Geometry: see drawing. Coordinates: mm, zero at the bounding-box minimum. Round coordinates to 2 decimals unless told otherwise and drop trailing zeros. Write each loop counter-clockwise with the first axis right and the second up, starting at its lowest first coordinate (ties: lowest second). Pieces come first, ordered by that corner, then holes. Notation, with made-up numbers: (-31, 89) -> (25, 89) arc R19 ccw to (25, 102) -> close; hole circle Ø4 at (67, -10.75). An arc over 180 degrees is marked (long way). Use CSV: the item, a comma, the result in double quotes.
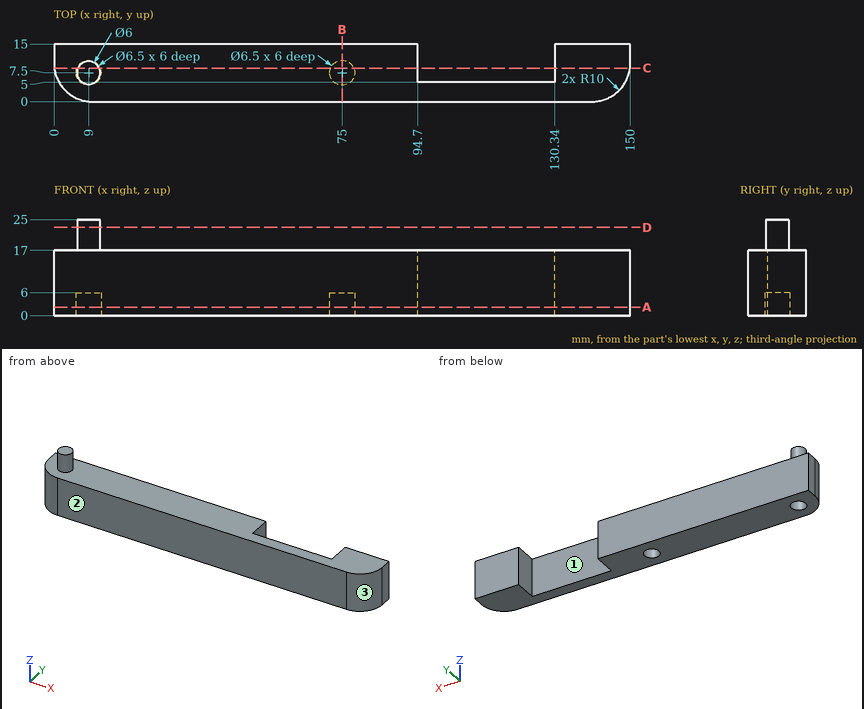
Item 1: Section query B-B on x = 75. Return the cut outline in (y, z).
Worked answers:
outline,"(0, 0) -> (4.25, 0) -> (4.25, 6) -> (10.75, 6) -> (10.75, 0) -> (15, 0) -> (15, 17) -> (0, 17) -> close"
Item 2: Section query D-D on z = 23. Return the cut outline in (x, y), plus the area to 3 significant figures.
Worked answers:
outline,"circle Ø6 at (9, 7.5)"
area,"28.3 mm²"
Item 3: Pull-direction query (X, two-part tool) for the marked faces 1, 2 and 3; classes: +X half, -X half, draft (parallel to the pull), parting line (faces both ways), or undercut.
Worked answers:
face 1,"undercut"
face 2,"draft"
face 3,"+X half"
Item 4: Section query A-A on z = 2.25. Return the cut outline in (x, y), plus the area to 3 significant figures.
Worked answers:
outline,"(0, 10) arc R10 ccw to (10, 0) -> (140, 0) arc R10 ccw to (150, 10) -> (150, 15) -> (130.34, 15) -> (130.34, 5) -> (94.7, 5) -> (94.7, 15) -> (0, 15) -> close; hole circle Ø6.5 at (9, 7.5); hole circle Ø6.5 at (75, 7.5)"
area,"1,780 mm²"
Item 5: Line query: line 1 (Y direction, x = 75, z = 1.6); line 2 (X direction, y = 12.75, z = 15.25); line 3 (Y direction, x = 9, z = 2.6). Output: solid intervals per line, ascending.
Worked answers:
line 1,"y = 0 to 4.25, 10.75 to 15"
line 2,"x = 0 to 94.7, 130.34 to 150"
line 3,"y = 0.05 to 4.25, 10.75 to 15"
Item 6: First-contact query: pin 1 Ø5 at (y, z) = (6.5, 19) entering from +X; pin 2 Ø2 at (x, y) = (8, 7) entering from -Z; pin 3 Ø8.5 at (x, y) = (75, 7.5) entering from +Z. Flat tips, straight axial feed; report the tip coordinate or a pass-through.
Worked answers:
pin 1,"stops at x = 149.8"
pin 2,"stops at z = 6"
pin 3,"stops at z = 17"
Item 7: Section query C-C on y = 8.75. Return the cut outline in (x, z).
Worked answers:
outline,"(0.08, 0) -> (6, 0) -> (6, 6) -> (12, 6) -> (12, 0) -> (72, 0) -> (72, 6) -> (78, 6) -> (78, 0) -> (94.7, 0) -> (94.7, 17) -> (11.73, 17) -> (11.73, 25) -> (6.27, 25) -> (6.27, 17) -> (0.08, 17) -> close; (130.34, 0) -> (149.92, 0) -> (149.92, 17) -> (130.34, 17) -> close"
